The listing builds one solid part. Answer for the finished solid, in the listing's coordinates (mm). A direction names the side the tool comes from. Round coordinates to 2 decimals unless told otherwise and drop trailing zeros. Write each loop counter-clockwise with the first axis right and the second up, starting at its lowest first coordinate (ties: lowest second). Pieces come first, ordered by that corner, then holes. Notation, with made-up numbers: (20.25, 83.5) - (41.25, 83.5) arc R10 cw to (41.25, 87.5) - close; hole circle Ø9 at (42.25, 52.25). An arc over 180 degrees is marked (long way). Return JSON: item names as keys, results as strings. Group by question number.
from build123d import *

# Parameters (mm, degrees)
F0_W     = 114.3
F0_H     = 50.8
F0_R     = 9.525
F1_DEPTH = 6.35
F2_W     = 34.29
F2_H     = 11.43
F3_DEPTH = 25.4
F4_W     = 53.34
F4_H     = 7.366
F5_DEPTH = 2.54


with BuildPart() as f1:
    # F0 (on Top) → F1 (new body)
    with BuildSketch(Plane.XY):
        with Locations((-57.15, 25.4)):
            Rectangle(F0_W, F0_H)
        with Locations((-96.52, 25.4)):
            Circle(F0_R, mode=Mode.SUBTRACT)
    extrude(amount=F1_DEPTH)

    # F2 (on face) → F3 (cut)
    with BuildSketch(Plane.XY.offset(6.35)):
        with Locations((-33.02, 25.4)):
            Rectangle(F2_W, F2_H)
        with BuildLine():
            Line((-50.165, 19.685), (-50.165, 31.115))
            ThreePointArc((-50.165, 31.115), (-55.88, 25.4), (-50.165, 19.685))
        make_face()
        with BuildLine():
            ThreePointArc((-15.875, 19.685), (-10.16, 25.4), (-15.875, 31.115))
            Line((-15.875, 31.115), (-15.875, 19.685))
        make_face()
    extrude(amount=-F3_DEPTH, mode=Mode.SUBTRACT)

    # F4 (on face) → F5 (cut)
    with BuildSketch(Plane.XY.offset(6.35)):
        with Locations((-55.88, 25.4)):
            Rectangle(F4_W, F4_H)
    extrude(amount=-F5_DEPTH, mode=Mode.SUBTRACT)


solid = f1.part
(1) Find section D-D (y = 33.5). Write down the section's boundary in (x, z).
(2) A flat-ended cylindrical pin translates along its axis: pin 1 (3.5 mm diameter, centred on x = -70, y = 25.5, fed in from +Z). Find the tip coordinate at first contact, or state that the pin passes through.
(3) Find section B-B (x = -20). Write down the section's boundary in (y, z) (3 decimals).
(4) For faces 1 (the flat face through (-114.3, 25, 3)), 2 (the flat face through (-33, 31.115, 3)), 3 (the flat face through (-69, 21.717, 5)), determine the directions among +Z, -Z, +X, -X, +Y, -Y from which every point of the face is accessible in a straight line to the end or side of a thin tool.
(5) Determine the mould class of faces 4 (the flat face through (-33, 19.685, 3)), 5 (the flat face through (-58, 26, 0)), 6 (the flat face through (0, 25, 3)), 7 (the flat face through (-82.55, 25, 5)) for opening direction X: +X half, -X half, draft (parallel to the pull), parting line (faces both ways), or undercut.
(6) Consider line 1 (X direction, y = 25.5, z = 2.25); line 2 (Y direction, x = -82.5, z = 4); line 3 (Y direction, x = -96.52, z = 1.5) (3 decimals). Determine where each line is inside the solid, lowest interval first.
(7) Find section A-A (z = 2.75). Write down the section's boundary in (x, y) (3 decimals).
(8) Find section C-C (y = 25.4). Write down the section's boundary in (x, z) (3 decimals), plus the area to 3 significant figures.
Check sheet entries:
{
 "1": {"outline": "(-114.3, 0) - (-101.53, 0) - (-101.53, 6.35) - (-114.3, 6.35) - close; (-91.51, 0) - (0, 0) - (0, 6.35) - (-91.51, 6.35) - close"},
 "2": {"pin 1": "stops at z = 3.81"},
 "3": {"outline": "(0, 0) - (19.685, 0) - (19.685, 6.35) - (0, 6.35) - close; (31.115, 0) - (50.8, 0) - (50.8, 6.35) - (31.115, 6.35) - close"},
 "4": {"face 1": "+Z, -Z, -X, +Y, -Y", "face 2": "+Z, -Z", "face 3": "+Z"},
 "5": {"face 4": "undercut", "face 5": "draft", "face 6": "+X half", "face 7": "undercut"},
 "6": {"line 1": "x = -114.3 to -106.04, -87 to -55.88, -10.16 to 0", "line 2": "y = 0 to 21.72, 29.08 to 50.8", "line 3": "y = 0 to 15.875, 34.925 to 50.8"},
 "7": {"outline": "(-114.3, 0) - (0, 0) - (0, 50.8) - (-114.3, 50.8) - close; hole circle Ø19.05 at (-96.52, 25.4); hole (-50.165, 19.685) - (-15.875, 19.685) arc R5.715 ccw to (-15.875, 31.115) - (-50.165, 31.115) arc R5.715 ccw to start"},
 "8": {"outline": "(-114.3, 0) - (-106.045, 0) - (-106.045, 6.35) - (-114.3, 6.35) - close; (-86.995, 0) - (-55.88, 0) - (-55.88, 3.81) - (-82.55, 3.81) - (-82.55, 6.35) - (-86.995, 6.35) - close; (-10.16, 0) - (0, 0) - (0, 6.35) - (-10.16, 6.35) - close", "area": "247 mm^2"}
}
